Geometry: final body of the model. Coordinates: model frame, mm. A direction names the side the tool comes from. Give positions to 0.01 mm unless a question says otherwise; leave off trailing zeros. Order: outer loops, then holes, each group sorted by start corner. A loop starts at its lowest first (then second) coordinate and runs counter-clockwise, first axis right, second up. Notation, with made-up numbers: (54, 34.25) - (107, 34.25) arc R11 cw to (107, 39.25) - close; hole circle Ø1 at (20.5, -29). An arc over 180 degrees is marked (long way). One line per item, written item: value.
```python
from build123d import *

# Parameters (mm, degrees)
F0_W           = 34.0106
F0_H           = 29.9974
F1_DEPTH       = 43.6118
F4_D           = 2.7051
F4_DEPTH       = 15.0876
F4_TIP         = 0.8126940303
F4_ON_F2_D     = 2.7051
F4_ON_F2_DEPTH = 15.0876
F4_ON_F2_TIP   = 0.8126940303


with BuildPart() as f1:
    # F0 (on Top) → F1 (new body)
    with BuildSketch(Plane.XY):
        with Locations((1.7151954423, -3.7325670248)):
            Rectangle(F0_W, F0_H)
    extrude(amount=-F1_DEPTH)

    # F4
    with Locations(Plane(origin=(0, 0, -43.6118), x_dir=(1, 0, 0), z_dir=(0, 0, -1))):
        with Locations((-10.2795045577, 12.7338670235), (13.7204954423, 12.7338670235), (13.7204954423, -5.2661329765), (-10.2795045577, -5.2661329765)):
            Hole(F4_D / 2, depth=F4_DEPTH)
            with Locations((0, 0, -(F4_DEPTH + F4_TIP / 2))):  # 118° drill point
                Cone(0, F4_D / 2, F4_TIP, mode=Mode.SUBTRACT)

    # F4 on F2
    with Locations(Plane.XY):
        with Locations((-10.2795045577, 5.2661329765), (13.7204954423, 5.2661329765), (13.7204954423, -12.7338670235), (-10.2795045577, -12.7338670235)):
            Hole(F4_ON_F2_D / 2, depth=F4_ON_F2_DEPTH)
            with Locations((0, 0, -(F4_ON_F2_DEPTH + F4_ON_F2_TIP / 2))):  # 118° drill point
                Cone(0, F4_ON_F2_D / 2, F4_ON_F2_TIP, mode=Mode.SUBTRACT)


solid = f1.part
```
1) Set-up query: faces 5 (the face through (-10.103, 3.925, -35.962)), 6 (the face through (1, -4, -43.612)), 7 (the face through (-9.986, -14.054, -7.649)). Return all of +Z, -Z, +X, -X, +Y, -Y with unobstructed straight access to the full face (end or side cutting, diameter ignored); none if empty.
Answers below:
face 5: -Z
face 6: -Z, +X, -X, +Y, -Y
face 7: +Z
2) Section A-A, the plane z = -14. Return loops of the section in (x, y), then the cut area to 3 significant figures.
Answers below:
outline: (-15.29, -18.73) - (18.72, -18.73) - (18.72, 11.27) - (-15.29, 11.27) - close; hole circle Ø2.71 at (-10.28, -12.73); hole circle Ø2.71 at (-10.28, 5.27); hole circle Ø2.71 at (13.72, -12.73); hole circle Ø2.71 at (13.72, 5.27)
area: 997 mm^2
3) First-contact query: pin 1 (2.5 mm diameter, centred on x = -10.28, y = 5.27, fed in from -Z); pin 2 (2 mm diameter, centred on x = -10.28, y = 5.27, fed in from +Z). Flat tips, straight axial feed; report the tip coordinate or a pass-through.
Answers below:
pin 1: z = -28.46
pin 2: z = -15.3
4) Material intervals for line 1 along Y through (x, z) = (-11, -29.5), sorted ascending.
Answers below:
line 1: -18.73 to -13.88, -11.59 to 4.12, 6.41 to 11.27
5) Mould query, pull axis X, two halves, no side actions, for faces 1 (the face through (1, 11.266, -22)), 2 (the face through (-15.29, -4, -22)), 3 (the face through (18.72, -4, -22)), 4 (the face through (-10.45, 5.42, -15.76)). Classes: released by +X, released by -X, zero draft, split by the parting line, or undercut.
Answers below:
face 1: zero draft
face 2: released by -X
face 3: released by +X
face 4: undercut
